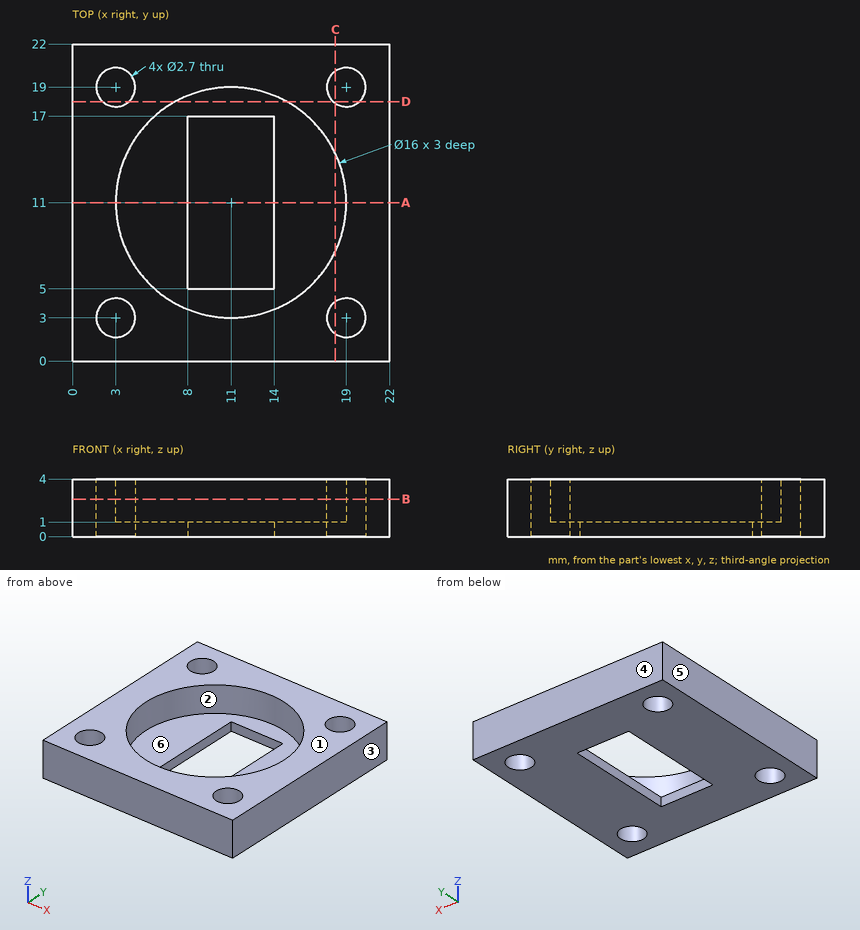
Check sheet for the drawn part. Datum: minimum x, y, z corner. Units: mm. A direction names the side the tool comes from. Round coordinates to 2 decimals unless told otherwise and drop trailing zeros. Order: outer loops, then holes, each group sorted by start corner. A loop starts at its lowest first (then second) coordinate and runs counter-clockwise, first axis right, second up.
(1) Access from +Z, -Z, +X, -X, +Y, -Y to the whole of each face (thin tool, end or side, straight path). Record for the marked faces 1 and 2.
(2) Cross-section at A-A, the plane y = 11. Enter the section's corners in (x, z).
(3) Scan lines: probe 1 along X at (y, z) = (7.5, 0.25); probe 2 along Y at (x, z) = (20, 3.7). Record each from-to range of solid material in increasing order.
(4) Go/stop test with flat-tipped pins: P1, Ø1, axis at y = 5, z = 1.5, coming from the -X side; P2, Ø2, axis at x = 12.5, y = 15, coming from the -Z side. Record where each tip stops, or that it passes through.
(5) Draft check along X on the marked faces 3, 4, 5 and 6. Enter one of: pulls with the +X half, pulls with the -X half, needs draft (parallel to the pull), parting line crosses it, or undercut.
(6) Cross-section at C-C, the plane x = 18.25. Enter the section's corners in (y, z), and give its area (3 significant figures).
(7) Cross-section at B-B, the plane z = 2.6. Enter the section's corners in (x, y).
(8) Cross-section at D-D, the plane y = 18. Enter the section's corners in (x, z).
Check sheet entries:
1. face 1: +Z, +X, -X, +Y, -Y
1. face 2: +Z
2. outline: (0, 0) - (8, 0) - (8, 1) - (3, 1) - (3, 4) - (0, 4) - close; (14, 0) - (22, 0) - (22, 4) - (19, 4) - (19, 1) - (14, 1) - close
3. probe 1: x = 0 to 8, 14 to 22
3. probe 2: y = 0 to 2.09, 3.91 to 18.09, 19.91 to 22
4. P1: stops at x = 0
4. P2: passes through
5. face 3: pulls with the +X half
5. face 4: needs draft
5. face 5: pulls with the -X half
5. face 6: undercut
6. outline: (0, 0) - (1.88, 0) - (1.88, 4) - (0, 4) - close; (4.12, 0) - (17.88, 0) - (17.88, 4) - (14.38, 4) - (14.38, 1) - (7.62, 1) - (7.62, 4) - (4.12, 4) - close; (20.12, 0) - (22, 0) - (22, 4) - (20.12, 4) - close
6. area: 49.7 mm2
7. outline: (0, 0) - (22, 0) - (22, 22) - (0, 22) - close; hole circle Ø2.7 at (3, 3); hole circle Ø2.7 at (3, 19); hole circle Ø16 at (11, 11); hole circle Ø2.7 at (19, 3); hole circle Ø2.7 at (19, 19)
8. outline: (0, 0) - (2.09, 0) - (2.09, 4) - (0, 4) - close; (3.91, 0) - (18.09, 0) - (18.09, 4) - (14.87, 4) - (14.87, 1) - (7.13, 1) - (7.13, 4) - (3.91, 4) - close; (19.91, 0) - (22, 0) - (22, 4) - (19.91, 4) - close
